Read the model definition and answer for the solid it produces. Units are mm, in the model's axes. A direction names the side the tool comes from. Round coordinates to 2 decimals unless told otherwise and drop trailing zeros. Loops run counter-clockwise (first coordinate to the right, second up) from the corner with the lowest first, then second, coordinate; pieces in that order, holes last. Notation, with made-up numbers: M 49.5,3.5 L 105.5,3.5 A13 ccw 105.5,14.5 Z; hole C 63,12 d6. An arc over 180 degrees is marked long. Answer as CSV lines item,"result".
```python
from build123d import *

# Parameters (mm, degrees)
SKETCH1_R           = 3
SKETCH1_R_2         = 4
BOSS_EXTRUDE1_DEPTH = 54
SKETCH2_W           = 34
SKETCH2_H           = 30
CUT_EXTRUDE1_DEPTH  = 54


with BuildPart() as part:
    # Sketch1 → Boss-Extrude1 (new body)
    with BuildSketch(Plane.XY):
        with BuildLine():
            Line((-59.598214286, 18), (-52.598214286, 25))
            Line((-52.598214286, 25), (87.401785714, 25))
            Line((87.401785714, 25), (90.401785714, 22))
            Line((90.401785714, 22), (90.401785714, 3))
            Line((90.401785714, 3), (87.401785714, 0))
            Line((87.401785714, 0), (-15.875401053, 0))
            ThreePointArc((-15.875401053, 0), (-25.133602051, -2.271894791), (-32.288437186, -8.571428571))
            ThreePointArc((-32.288437186, -8.571428571), (-49.090059313, -14.311650088), (-59.598214286, 0))
            Line((-59.598214286, 0), (-59.598214286, 18))
        make_face()
        with Locations((78.401785714, 12.5)):
            Circle(SKETCH1_R, mode=Mode.SUBTRACT)
        with Locations((32.901785714, 12.5)):
            Circle(SKETCH1_R_2, mode=Mode.SUBTRACT)
    extrude(amount=BOSS_EXTRUDE1_DEPTH)

    # Sketch2 → Cut-Extrude1 (cut)
    with BuildSketch(Plane(origin=(0, 25, 0), x_dir=(1, 0, 0), z_dir=(0, 1, 0))):
        with Locations((73.401785714, -27)):
            Rectangle(SKETCH2_W, SKETCH2_H)
    extrude(amount=-CUT_EXTRUDE1_DEPTH, mode=Mode.SUBTRACT)


solid = part.part
```
1) A tool of negligible diameter and unlimited length cuts with its end or side. For faces 1 (the cylindrical face through (-48.8, -14.4, 26.6)), 2 (the flat face through (25, 0, 27)), 3 (the flat face through (73, 13, 12)), from which of +Z, -Z, +X, -X, +Y, -Y can it reach the whole face along a straight path? Write none if from no direction.
Evaluation:
face 1,"+Z, -Z, -Y"
face 2,"+Z, -Z, +X, -Y"
face 3,"+X, +Y, -Y"
2) Each of these flat-tipped pins is pushed along its axis until it touches: P1, Ø10, axis at x = 16, z = 48.5, coming from the -Y side; P2, Ø10, axis at y = -10.5, z = 11, coming from the -X side; P3, Ø8, axis at y = -8.5, z = 19, coming from the -X side. Where does it stop, or does it pass through?
Evaluation:
P1,"stops at y = 0"
P2,"stops at x = -58.55"
P3,"stops at x = -58.91"
3) Find section D-D, the plane z = 38. Give the vertices of the cut face in (x, y).
Evaluation:
outline,"M -59.6,0 A15 ccw -32.29,-8.57 A20 cw -15.88,0 L 56.4,0 L 56.4,25 L -52.6,25 L -59.6,18 Z; hole C 32.9,12.5 d8"
4) Determine the mould class of faces 4 (the cylindrical face through (75.405, 12.632, 5.916)), 5 (the cylindrical face through (75.405, 12.632, 47.916)), 6 (the flat face through (73, 13, 42)), 7 (the flat face through (90.402, 13, 48)) for opening direction X: released by +X, released by -X, zero draft, split by the parting line, or undercut.
Evaluation:
face 4,"undercut"
face 5,"undercut"
face 6,"zero draft"
face 7,"released by +X"
5) Find section C-C, the plane x = 32. Give the vertices of the cut face in (y, z).
Evaluation:
outline,"M 0,0 L 8.6,0 L 8.6,54 L 0,54 Z; M 16.4,0 L 25,0 L 25,54 L 16.4,54 Z"
6) Straight lines are drawn through the part: line 1 (X direction, y = 12, z = 19); line 2 (X direction, y = 12, z = 48); line 3 (Y direction, x = 61.5, z = 47). For each, find the intervals that lie inside material, in ascending order.
Evaluation:
line 1,"x = -59.6 to 28.93, 36.87 to 56.4"
line 2,"x = -59.6 to 28.93, 36.87 to 75.44, 81.36 to 90.4"
line 3,"y = 0 to 25"
7) Find section A-A, the plane z = 48.5. Give the vertices of the cut face in (x, y).
Evaluation:
outline,"M -59.6,0 A15 ccw -32.29,-8.57 A20 cw -15.88,0 L 87.4,0 L 90.4,3 L 90.4,22 L 87.4,25 L -52.6,25 L -59.6,18 Z; hole C 32.9,12.5 d8; hole C 78.4,12.5 d6"
8) Find section B-B, the plane y = 12.5. Give the vertices of the cut face in (x, z).
Evaluation:
outline,"M -59.6,0 L 28.9,0 L 28.9,54 L -59.6,54 Z; M 36.9,0 L 75.4,0 L 75.4,12 L 56.4,12 L 56.4,42 L 75.4,42 L 75.4,54 L 36.9,54 Z; M 81.4,0 L 90.4,0 L 90.4,12 L 81.4,12 Z; M 81.4,42 L 90.4,42 L 90.4,54 L 81.4,54 Z"
